Geometry check sheet. Reference: the model listing, model coordinates, mm. A direction names the side the tool comes from. Coordinates: 2 decimals unless noted, no trailing zeros. Write each loop counter-clockwise with the first axis right and the second up, starting at its lowest first coordinate (ties: lowest second). Pieces come first, ordered by that corner, then holes.
from build123d import *

# Parameters (mm, degrees)
SKETCH1_R           = 40
BOSS_EXTRUDE1_DEPTH = 10
BOSS_EXTRUDE1_TAPER = 30
SKETCH2_W           = 38.335841008
SKETCH2_H           = 10.708335478
BOSS_EXTRUDE2_DEPTH = 60
SKETCH3_R           = 19.167920504
BOSS_EXTRUDE3_DEPTH = 20


with BuildPart() as part:
    # Sketch1 → Boss-Extrude1 (new body)
    with BuildSketch(Plane(origin=(0, 0, 0), x_dir=(1, 0, 0), z_dir=(0, 1, 0))):
        Circle(SKETCH1_R)
    extrude(amount=BOSS_EXTRUDE1_DEPTH, taper=BOSS_EXTRUDE1_TAPER)

    # Sketch2 → Boss-Extrude2 (add)
    with BuildSketch(Plane(origin=(0, 10, 0), x_dir=(1, 0, 0), z_dir=(0, 1, 0))):
        Rectangle(SKETCH2_W, SKETCH2_H)
    extrude(amount=BOSS_EXTRUDE2_DEPTH)

    # Sketch3 → Boss-Extrude3 (add)
    with BuildSketch(Plane(origin=(0, 0, -5.354167739), x_dir=(-1, 0, 0), z_dir=(0, 0, -1))):
        with Locations((0, 70)):
            Circle(SKETCH3_R)
    extrude(amount=-BOSS_EXTRUDE3_DEPTH)


solid = part.part
1. Thickness scan on line 1 along Z through (x, y) = (-5, 52); line 2 along Y through (x, z) = (7, 8); line 3 along Y through (x, z) = (-9.5, 21.5). Record the ranges inside material, lowest first.
Computed values:
line 1: z = -5.35 to 14.65
line 2: y = 0 to 10, 52.16 to 87.84
line 3: y = 0 to 10
2. Sectioned sample at A-A, the plane x = 0. Record the boundary of the cut face in (y, z), and give its area (3 significant figures).
Computed values:
outline: (0, -40) - (10, -34.23) - (10, -5.35) - (89.17, -5.35) - (89.17, 14.65) - (50.83, 14.65) - (50.83, 5.35) - (10, 5.35) - (10, 34.23) - (0, 40) - close
area: 1,950 mm2
3. Sectioned sample at C-C, the plane y = 13. Record the boundary of the cut face in (x, z), and give its area (3 significant figures).
Computed values:
outline: (-19.17, -5.35) - (19.17, -5.35) - (19.17, 5.35) - (-19.17, 5.35) - close
area: 411 mm2
4. Gauge pin test, flat ends, axial feed: pin 1 Ø12 at (x, y) = (18, 70.5) entering from +Z; pin 2 Ø3 at (y, z) = (32, 0) entering from -X; pin 3 Ø19 at (x, y) = (-1.5, 35) entering from -Z. Record the tip position at first contact, or that the pin passes through.
Computed values:
pin 1: stops at z = 14.65
pin 2: stops at x = -19.17
pin 3: stops at z = -5.35
5. Sectioned sample at D-D, the plane y = 72.5. Record the boundary of the cut face in (x, z).
Computed values:
outline: (-19, -5.35) - (19, -5.35) - (19, 14.65) - (-19, 14.65) - close
6. Access from +Z, -Z, +X, -X, +Y, -Y to the whole of each face (thin tool, end or side, straight path). Record for faces 4 (the flat face through (19.168, 40, 0)), 5 (the conical face through (32.913, 9.514, -10.365)), 6 (the flat face through (0, 49, -5.354)), 7 (the flat face through (-19.168, 40, 0)).
Computed values:
face 4: +Z, -Z, +X, +Y
face 5: +Y
face 6: -Z, +X, -X, +Y
face 7: +Z, -Z, -X, +Y
7. Sectioned sample at B-B, the plane y = 55. Record the boundary of the cut face in (x, z).
Computed values:
outline: (-19.17, -5.35) - (19.17, -5.35) - (19.17, 5.35) - (11.93, 5.35) - (11.93, 14.65) - (-11.93, 14.65) - (-11.93, 5.35) - (-19.17, 5.35) - close
8. Draft check along Y on faces 1 (the flat face through (0, 70, 14.646)), 2 (the flat face through (-1, 0, -1)), 3 (the cylindrical face through (2.495, 89.005, 6.728)). Enter one of: released by +Y, released by -Y, zero draft, split by the parting line, or undercut.
Computed values:
face 1: zero draft
face 2: released by -Y
face 3: undercut
